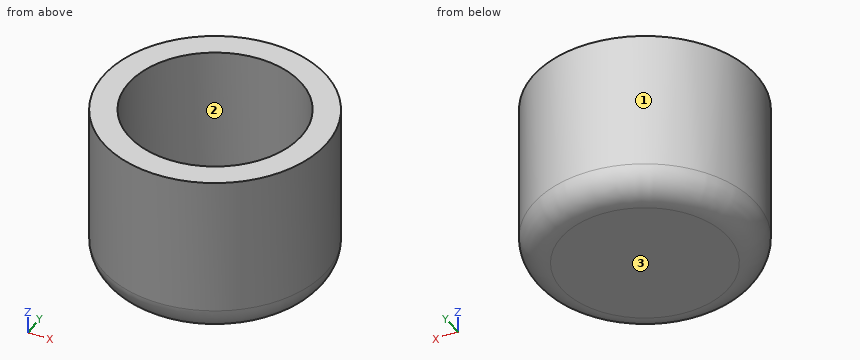
```python
from build123d import *

# Parameters (mm, degrees)
CYLINDER_R     = 8
CYLINDER_DEPTH = 12
SKETCH_R       = 6.2
POCKET_DEPTH   = 10
FILLET_R       = 2


with BuildPart() as part:
    # Cylinder → Cylinder (new body)
    with BuildSketch(Plane.XY):
        Circle(CYLINDER_R)
    extrude(amount=CYLINDER_DEPTH)

    # Sketch → Pocket (cut)
    with BuildSketch(Plane.XY.offset(12)):
        Circle(SKETCH_R)
    extrude(amount=-POCKET_DEPTH, mode=Mode.SUBTRACT)

    # Fillet
    fillet_edges = [part.edges().sort_by_distance(p)[0] for p in [
        (-8, 0, 0),
    ]]
    fillet(fillet_edges, radius=FILLET_R)


solid = part.part
```
Input: part model. Units: mm. Frame: model coordinates. Face numbers are marked on the shaded views. Round coordinates to 2 decimals unless told otherwise and drop trailing zeros. Loops run counter-clockwise (first coordinate to the right, second up) from the corner with the lowest first, then second, coordinate; pieces in that order, holes last. Notation, with made-up numbers: M -18,12.25 L 33,12.25 A7 ccw 33,25.25 Z; hole C 45.5,-1.75 d8. An arc over 180 degrees is marked long. Answer in a Markdown table with one row per item. Add a question column.
1. Section A-A (y = 0). Output: boundary loops of the cut face in (x, z).
2. Contact query for flat-ended pins moving along their axis: pin 1 (1.5 mm diameter, centred on x = 5, z = 6, fed in from +Y); pin 2 (3 mm diameter, centred on x = -4, z = 3.5, fed in from -Y); pin 3 (3 mm diameter, centred on x = 5.5, z = 8, fed in from +Y). Output: stop coordinate, or through.
3. Section B-B (z = 5.75). Output: boundary loops of the cut face in (x, y), and give its area (3 significant figures).
4. Mould query, pull axis Y, two halves, no side actions, for the marked faces 1, 2 and 3. Classes: released by +Y, released by -Y, zero draft, split by the parting line, or undercut.
5. Ray query, probe 1 along Y at (x, z) = (0, 6.5); probe 2 along Z at (x, y) = (-1, -0.25); probe 3 along X at (y, z) = (-1.5, 6.25). Return the intervals inside material, ascending.
Values follow:
| question | item | result |
|---|---|---|
| 1 | outline | M -8,2 A2 ccw -6,0 L 6,0 A2 ccw 8,2 L 8,12 L 6.2,12 L 6.2,2 L -6.2,2 L -6.2,12 L -8,12 Z |
| 2 | pin 1 | y = 6.78 |
| 2 | pin 2 | y = -7.6 |
| 2 | pin 3 | y = 6.93 |
| 3 | outline | C 0,0 d16; hole C 0,0 d12.4 |
| 3 | area | 80.3 mm^2 |
| 4 | face 1 | split by the parting line |
| 4 | face 2 | undercut |
| 4 | face 3 | zero draft |
| 5 | probe 1 | -8 to -6.2, 6.2 to 8 |
| 5 | probe 2 | 0 to 2 |
| 5 | probe 3 | -7.86 to -6.02, 6.02 to 7.86 |
